Build history of the part. All positions in model axes, mm. A direction names the side the tool comes from. Round coordinates to 2 decimals unless told otherwise and drop trailing zeros. Order: outer loops, then holes, each group sorted by start corner. A loop starts at its lowest first (then second) coordinate and runs counter-clockwise, first axis right, second up. Notation, with made-up numbers: (25, 33) -> (37, 33) arc R32 cw to (37, 60) -> close; hole circle Ø2 at (-6, -25.5). An arc over 180 degrees is marked (long way). Write item = value, one per line.
from build123d import *

# Parameters (mm, degrees)
F2_R        = 3.2512
F3_SIZE2    = 2.54
F3_SIZE     = 2.54
F4_S5_R     = 1.5875
F4_T6_DEPTH = 6
F5_R        = 2.4384


# Not quite as in the source:
# - a fillet or chamfer that OpenCascade refuses, or shapes differently, is made with other operations: its cross-section is extruded or revolved along the edge and cut away or added


with BuildPart() as f1:
    # F0 (on Front) → F1 (revolve)
    with BuildSketch(Plane.XZ):
        Polygon((-50.8, 0), (0, 0), (0, 3.175), (-6.35, 3.175), (-6.35, 1.5875), (-7.9502, 1.5875), (-7.9502, 3.175), (-47.625, 3.175), (-47.625, 19.05), (-50.8, 19.05), align=None)
    revolve(axis=Axis((-25.4, 0, 0), (1, 0, 0)))

    # F2
    f2_edges = [f1.edges().sort_by_distance(p)[0] for p in [
        (-47.625, 0, -3.175),
    ]]
    fillet(f2_edges, radius=F2_R)

    # F3
    f3_edges = [f1.edges().sort_by_distance(p)[0] for p in [
        (-47.625, 0, -6.4262),
        (-47.625, 0, -19.05),
    ]]
    chamfer(f3_edges, length=F3_SIZE, length2=F3_SIZE2)

    # F4: chamfer of 1.6002 on 1 edges, made by hand


with BuildPart() as f4_tool2:
    # F4_s3 → F4_t4 (revolve)
    with BuildSketch(Plane.XZ):
        Polygon((-9.5504, 3.175), (-7.9502, 1.5748), (-7.9502, 3.175), align=None)
    revolve(axis=Axis((-7.9502, 0, 0), (1, 0, 0)))

    # F4_s5 → F4_t6 (cut, symmetric)
    with BuildSketch(Plane.YZ.offset(-8.8)):
        Circle(F4_S5_R)
    extrude(amount=F4_T6_DEPTH, both=True, mode=Mode.SUBTRACT)


with BuildPart() as f1_1:
    add(f1.part)

    # F4_t1: cut F4_tool2
    add(f4_tool2.part, mode=Mode.SUBTRACT)

    # F5
    f5_edges = [f1_1.edges().sort_by_distance(p)[0] for p in [
        (0, 0, -3.175),
    ]]
    fillet(f5_edges, radius=F5_R)


solid = f1_1.part
Q1. Flat gauge pins, fed straight in: pin 1 (6 mm diameter, centred on y = 6, z = -3.5, fed in from +X); pin 2 (6 mm diameter, centred on x = -37, z = 5, fed in from -Y); pin 3 (8 mm diameter, centred on x = -44, z = 10, fed in from +Y). Where does each tip first touch, or does it go through?
Check values:
pin_1 = -46.48
pin_2 = -2.47
pin_3 = 14.27
Q2. Probe probe 1 along X at (y, z) = (12, 6) (3 decimals); probe 2 along Y at (x, z) = (-48, 2); probe 3 along Z at (x, y) = (-48, -6.5). List the from-to ranges inside material, lowest first.
Check values:
probe_1 = -50.8 to -47.625
probe_2 = -16.77 to 16.77
probe_3 = -15.58 to 15.58
Q3. Mould opens along X. For faces 1 (the face through (-6.35, 1.4, 1.4)), 2 (the face through (-27.21, 3.1, -0.69)), 3 (the face through (0, 0, 0)), 4 (the face through (-50.8, 0, 0)) say: released by +X, released by -X, zero draft, split by the parting line, or undercut.
Check values:
face_1 = undercut
face_2 = zero draft
face_3 = released by +X
face_4 = released by -X
Q4. Cut at A-A, the plane x = -25. List the corners of the cut face in (y, z) (3 decimals).
Check values:
outline = circle Ø6.35 at (0, 0)
Q5. Cut at B-B, the plane x = -45.5. List the corners of the cut face in (y, z), and give its area (3 significant figures).
Check values:
outline = circle Ø6.75 at (0, 0)
area = 35.8 mm²
Q6. Which spindle directions (+Z, -Z, +X, -X, +Y, -Y) get a long thin tool onto all of the face, cutting with end or side? Do faces 5 (the face through (-50.49, 11.59, -15.12)), 6 (the face through (-47.625, 7, 0)). Say none if no direction does.
Check values:
face_5 = +X, -X
face_6 = +X
